Can you work these out from the model? Positions are in its coordinate system, mm. Face numbers are marked on the shaded views. A direction names the side the tool comes from. Give positions to 0.01 mm unless a question says otherwise; leave off trailing zeros. Write each loop counter-clockwise with the first axis right and the second up, starting at its lowest first coordinate (ties: lowest second). Pieces come first, ordered by that corner, then holes.
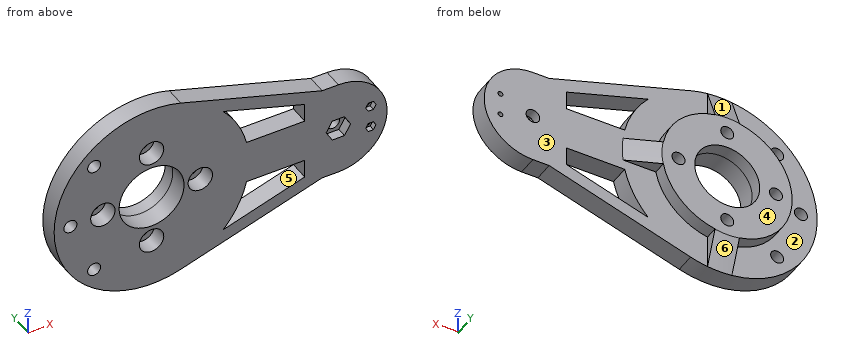
from build123d import *
from OCP.BRepFilletAPI import BRepFilletAPI_MakeChamfer
from build123d.topology import SkipClean

# Parameters (mm, degrees)
SKETCH1_R           = 40
SKETCH1_R_2         = 20
BOSS_EXTRUDE1_DEPTH = 8
BOSS_EXTRUDE2_START = 12
SKETCH3_R           = 20
BOSS_EXTRUDE2_DEPTH = 12
SKETCH5_R           = 7.5
CUT_EXTRUDE3_DEPTH  = 10
SKETCH2_R           = 4
CUT_EXTRUDE1_DEPTH  = 20
BOSS_EXTRUDE3_DEPTH = 8
CHAMFER1_SIZE       = 19.800694827
CHAMFER1_SIZE_2     = 8
BOSS_EXTRUDE4_DEPTH = 12
CUT_EXTRUDE4_DEPTH  = 6
SKETCH9_R           = 4.2
CUT_EXTRUDE5_DEPTH  = 6
CUT_EXTRUDE7_START  = -12
CUT_EXTRUDE7_DEPTH  = 12
SKETCH_1_R          = 4
CUT_EXTRUDE_1_DEPTH = 158.381701605
SKETCH_2_R          = 1.5
CUT_EXTRUDE_2_DEPTH = 158.381701605
CUT_EXTRUDE_3_DEPTH = 3.5
SKETCH_1_4_R        = 4
CUT_EXTRUDE_4_DEPTH = 158.381701605


with BuildPart() as part:
    # Sketch1 → Boss-Extrude1 (new body)
    with BuildSketch(Plane(origin=(0, 0, 0), x_dir=(1, 0, 0), z_dir=(0, 1, 0))):
        with Locations(Location((0, 0, 0), (0, 0, 270))):
            Circle(SKETCH1_R)
        with Locations(Location((0, 0, 0), (0, 0, 270))):
            Circle(SKETCH1_R_2, mode=Mode.SUBTRACT)
    extrude(amount=BOSS_EXTRUDE1_DEPTH)

    # Sketch3 → Boss-Extrude2 (add)
    with SkipClean():  # the faces are left unmerged after this step: merging them gives an invalid solid
        with BuildSketch(Plane.XZ.offset(BOSS_EXTRUDE2_START)):
            with BuildLine():
                Line((17.925820686, 57.259627599), (105, 30))
                Line((105, 30), (105, -30))
                Line((105, -30), (17.925820686, -57.259627599))
                ThreePointArc((17.925820686, -57.259627599), (-60, 0), (17.925820686, 57.259627599))
            make_face()
            with Locations(Location((0, 0, 0), (0, 0, 270))):
                Circle(SKETCH3_R, mode=Mode.SUBTRACT)
        extrude(amount=-BOSS_EXTRUDE2_DEPTH)

    # Sketch5 → Cut-Extrude3 (cut)
    with SkipClean():  # the faces are left unmerged after this step: merging them gives an invalid solid
        with BuildSketch(Plane.XZ.offset(12)):
            with Locations(Location((0, 30, 0), (0, 0, 270))):
                Circle(SKETCH5_R)
            with Locations(Location((30, 0, 0), (0, 0, 270))):
                Circle(SKETCH5_R)
            with Locations(Location((0, -30, 0), (0, 0, 270))):
                Circle(SKETCH5_R)
            with Locations(Location((-30, 0, 0), (0, 0, 270))):
                Circle(SKETCH5_R)
        extrude(amount=-CUT_EXTRUDE3_DEPTH, mode=Mode.SUBTRACT)

    # Sketch2 → Cut-Extrude1 (cut)
    with SkipClean():  # the faces are left unmerged after this step: merging them gives an invalid solid
        with BuildSketch(Plane(origin=(0, 8, 0), x_dir=(1, 0, 0), z_dir=(0, 1, 0))):
            with Locations(Location((30, 0, 0), (0, 0, 270))):
                Circle(SKETCH2_R)
            with Locations(Location((0, -30, 0), (0, 0, 270))):
                Circle(SKETCH2_R)
            with Locations(Location((-30, 0, 0), (0, 0, 270))):
                Circle(SKETCH2_R)
            with Locations(Location((0, 30, 0), (0, 0, 270))):
                Circle(SKETCH2_R)
        extrude(amount=-CUT_EXTRUDE1_DEPTH, mode=Mode.SUBTRACT)

    # Sketch6 → Boss-Extrude3 (add)
    with SkipClean():  # the faces are left unmerged after this step: merging them gives an invalid solid
        with BuildSketch(Plane(origin=(0, 0, 0), x_dir=(1, 0, 0), z_dir=(0, 1, 0))):
            with BuildLine():
                Line((-7.5, -39.290584114), (-7.5, -59.529404499))
                ThreePointArc((-7.5, -59.529404499), (0, -60), (7.5, -59.529404499))
                Line((7.5, -59.529404499), (7.5, -39.290584114))
                ThreePointArc((7.5, -39.290584114), (0, -40), (-7.5, -39.290584114))
            make_face()
            with BuildLine():
                Line((-7.5, 39.290584114), (-7.5, 59.529404499))
                ThreePointArc((-7.5, 59.529404499), (0, 60), (7.5, 59.529404499))
                Line((7.5, 59.529404499), (7.5, 39.290584114))
                ThreePointArc((7.5, 39.290584114), (0, 40), (-7.5, 39.290584114))
            make_face()
            with BuildLine():
                Line((39.290584114, 7.5), (59.529404499, 7.5))
                ThreePointArc((59.529404499, 7.5), (60, 0), (59.529404499, -7.5))
                Line((59.529404499, -7.5), (39.290584114, -7.5))
                ThreePointArc((39.290584114, -7.5), (40, 0), (39.290584114, 7.5))
            make_face()
        extrude(amount=BOSS_EXTRUDE3_DEPTH)

    # Chamfer1
    chamfer1_edges_1 = [part.edges().sort_by_distance(p)[0] for p in [
        (0, 8, -60),
    ]]
    chamfer1_side_1 = [part.faces().sort_by_distance(p)[0] for p in [
        (0, 8, -59.84),
    ]]
    chamfer1_edges_2 = [part.edges().sort_by_distance(p)[0] for p in [
        (60, 8, 0),
    ]]
    chamfer1_side_2 = [part.faces().sort_by_distance(p)[0] for p in [
        (60, 7.84, 0),
    ]]
    chamfer1_edges_3 = [part.edges().sort_by_distance(p)[0] for p in [
        (0, 8, 60),
    ]]
    chamfer1_side_3 = [part.faces().sort_by_distance(p)[0] for p in [
        (0, 8, 59.84),
    ]]
    chamfer1 = BRepFilletAPI_MakeChamfer(part.part.solid().wrapped)
    for e in chamfer1_edges_1:
        chamfer1.Add(CHAMFER1_SIZE - 0.0001, CHAMFER1_SIZE_2 - 0.0001, e.wrapped, chamfer1_side_1[0].wrapped)
    for e in chamfer1_edges_2:
        chamfer1.Add(CHAMFER1_SIZE_2 - 0.0001, CHAMFER1_SIZE - 0.0001, e.wrapped, chamfer1_side_2[0].wrapped)
    for e in chamfer1_edges_3:
        chamfer1.Add(CHAMFER1_SIZE - 0.0001, CHAMFER1_SIZE_2 - 0.0001, e.wrapped, chamfer1_side_3[0].wrapped)
    add(Compound.cast(chamfer1.Shape()), mode=Mode.REPLACE)  # a hair under: the kernel refuses the full size

    # Sketch7 → Boss-Extrude4 (add)
    with BuildSketch(Plane.XZ.offset(12)):
        with BuildLine():
            Line((115, 30), (105, 30))
            Line((105, 30), (105, -30))
            Line((105, -30), (115, -30))
            ThreePointArc((115, -30), (145, 0), (115, 30))
        make_face()
    extrude(amount=-BOSS_EXTRUDE4_DEPTH)

    # Sketch8 → Cut-Extrude4 (cut)
    with BuildSketch(Plane.XZ.offset(12)):
        Polygon((111.24722325, -6.5), (118.75277675, -6.5), (122.505553499, 0), (118.75277675, 6.5), (111.24722325, 6.5), (107.494446501, 0), align=None)
    extrude(amount=-CUT_EXTRUDE4_DEPTH, mode=Mode.SUBTRACT)

    # Sketch9 → Cut-Extrude5 (cut)
    with BuildSketch(Plane.XZ.offset(6)):
        with Locations(Location((115, 0, 0), (0, 0, 270))):
            Circle(SKETCH9_R)
    extrude(amount=-CUT_EXTRUDE5_DEPTH, mode=Mode.SUBTRACT)

    # Sketch11 → Cut-Extrude7 (cut)
    with BuildSketch(Plane(origin=(0, 0, 0), x_dir=(1, 0, 0), z_dir=(0, 1, 0)).offset(CUT_EXTRUDE7_START)):
        with BuildLine():
            Line((94.268829829, 24.976653188), (94.268829829, 13.5))
            Line((94.268829829, 13.5), (58.46152581, 13.5))
            ThreePointArc((58.46152581, 13.5), (53.052110577, 28.026301278), (44.101832404, 40.682040001))
            Line((44.101832404, 40.682040001), (94.268829829, 24.976653188))
        make_face()
    cut_extrude7 = extrude(amount=CUT_EXTRUDE7_DEPTH, mode=Mode.SUBTRACT)

    # Mirror1: Cut-Extrude7 across plane
    add(cut_extrude7.mirror(Plane.XY), mode=Mode.SUBTRACT)

    # 草图1 → 切除-拉伸1 (cut, through all)
    with BuildSketch(Plane(origin=(0, 0, 0), x_dir=(1, 0, 0), z_dir=(0, 1, 0))):
        with Locations(Location((-35.355339059, 35.355339059, 0), (0, 0, 270))):
            Circle(SKETCH_1_R)
        with Locations(Location((-35.355339059, -35.355339059, 0), (0, 0, 270))):
            Circle(SKETCH_1_R)
    extrude(amount=-CUT_EXTRUDE_1_DEPTH, mode=Mode.SUBTRACT)

    # 草图2 → 切除-拉伸2 (cut, through all)
    with BuildSketch(Plane(origin=(0, 0, 0), x_dir=(1, 0, 0), z_dir=(0, 1, 0))):
        with Locations(Location((135, -7, 0), (0, 0, 270))):
            Circle(SKETCH_2_R)
        with Locations(Location((135, 7, 0), (0, 0, 270))):
            Circle(SKETCH_2_R)
    extrude(amount=-CUT_EXTRUDE_2_DEPTH, mode=Mode.SUBTRACT)

    # 草图3 → 切除-拉伸3 (cut)
    with BuildSketch(Plane.XZ.offset(12)):
        Polygon((133.41228676, -9.75), (136.58771324, -9.75), (138.175426481, -7), (136.58771324, -4.25), (133.41228676, -4.25), (131.824573519, -7), align=None)
        Polygon((133.41228676, 4.25), (136.58771324, 4.25), (138.175426481, 7), (136.58771324, 9.75), (133.41228676, 9.75), (131.824573519, 7), align=None)
    extrude(amount=-CUT_EXTRUDE_3_DEPTH, mode=Mode.SUBTRACT)

    # 草图1<4> → 切除-拉伸4 (cut, through all)
    with BuildSketch(Plane(origin=(0, 0, 0), x_dir=(1, 0, 0), z_dir=(0, 1, 0))):
        with Locations(Location((-35.355339059, 35.355339059, 0), (0, 0, 270))):
            Circle(SKETCH_1_4_R)
        with Locations(Location((-35.355339059, -35.355339059, 0), (0, 0, 270))):
            Circle(SKETCH_1_4_R)
        with Locations(Location((-50, -0.068188384, 0), (0, 0, 270))):
            Circle(SKETCH_1_4_R)
    extrude(amount=-CUT_EXTRUDE_4_DEPTH, mode=Mode.SUBTRACT)


solid = part.part
(1) Will these pins go through, and if not, where does the flat tip stop? P1, Ø4, axis at x = 135, z = -7, coming from the +Y side; P2, Ø12, axis at x = 27, y = -5.5, coming from the -Z side; P3, Ø12, axis at x = 100, z = -32, coming from the -Y side; P4, Ø2, axis at x = -32, y = -3.5, coming from the -Z side.
Returned:
P1: stops at y = 0
P2: stops at z = -56.3
P3: stops at y = -12
P4: stops at z = -51.37
(2) If we mould it in two halves opening along X, with no side actions, what happens to the marked faces 4, 5 and 6? For each: +X half, -X half, draft (parallel to the pull), parting line (faces both ways), or undercut.
Returned:
face 4: draft
face 5: undercut
face 6: parting line
(3) Imagine slicing it at C-C, the plane x = -11.5. Write out the boundary of the cut face in (y, z), plus the area to 3 significant figures.
Returned:
outline: (-12, -58.89) - (0, -58.89) - (0, -38.31) - (8, -38.31) - (8, -16.36) - (-12, -16.36) - close; (-12, 16.36) - (8, 16.36) - (8, 38.31) - (0, 38.31) - (0, 58.89) - (-12, 58.89) - close
area: 1,370 mm2
(4) Imagine slicing it at A-A, the plane x = 66. Write out the boundary of the cut face in (y, z), plus the area to 3 significant figures.
Returned:
outline: (-12, -42.21) - (0, -42.21) - (0, -33.83) - (-12, -33.83) - close; (-12, -13.5) - (0, -13.5) - (0, 13.5) - (-12, 13.5) - close; (-12, 33.83) - (0, 33.83) - (0, 42.21) - (-12, 42.21) - close
area: 525 mm2
(5) For the marked faces 1, 2 and 3, which set-ups out of +Z, -Z, +X, -X, +Y, -Y let a thin tool reach every point of the face, with its end or its side?
Returned:
face 1: +Z, +Y
face 2: -X, +Y
face 3: +X, +Y
(6) Imagine slicing it at D-D, the plane x = -50. Write out the boundary of the cut face in (y, z), plus the area to 3 significant figures.
Returned:
outline: (-12, -33.17) - (0, -33.17) - (0, -3.93) - (-12, -3.93) - close; (-12, 4.07) - (0, 4.07) - (0, 33.17) - (-12, 33.17) - close
area: 700 mm2
(7) Imagine slicing it at B-B, the plane y = 2. Write out the boundary of the cut face in (x, z).
Returned:
outline: (-7.5, -54.54) arc R55.05 ccw to (7.5, -54.54) - (7.5, -39.29) arc R40 ccw to (39.29, -7.5) - (54.54, -7.5) arc R55.05 ccw to (54.54, 7.5) - (39.29, 7.5) arc R40 ccw to (7.5, 39.29) - (7.5, 54.54) arc R55.05 ccw to (-7.5, 54.54) - (-7.5, 39.29) arc R40 ccw to (-7.5, -39.29) - close; hole circle Ø8 at (-30, 0); hole circle Ø40 at (0, 0); hole circle Ø8 at (0, -30); hole circle Ø8 at (0, 30); hole circle Ø8 at (30, 0)
(8) If I drill on L1, parallel to Z at x = 135, y = -5.5; L2, parallel to Z at x = 105, y = -9; L3, parallel to Z at x = 54, y = -5.75, over which ranges is the centre line in solid material (lowest first)?
Returned:
L1: z = -22.36 to -8.5, -5.5 to 5.5, 8.5 to 22.36
L2: z = -30 to 30
L3: z = -45.97 to -37.58, -26.15 to 26.15, 37.58 to 45.97
